from build123d import *

# Parameters (mm, degrees)
SKETCH_2_R               = 25
EXTRUDE_1_DEPTH          = 6
SKETCH_3_R               = 30
EXTRUDE_2_DEPTH          = 2
EXTRUDE_START            = 2
SKETCH_4_R               = 30
EXTRUDE_4_DEPTH          = 2
CUT_EXTRUDE_1_DEPTH      = 44.588989435
CUT_EXTRUDE_1_DEPTH_BACK = 44.588989435
SKETCH_5_R               = 20
CUT_EXTRUDE_3_DEPTH      = 44.588989435
CUT_EXTRUDE_3_DEPTH_BACK = 44.588989435
SKETCH_7_R               = 1.25


with BuildPart() as part:
    # 스케치2 → 보스-돌출1 (new body)
    with BuildSketch(Plane.XY):
        Circle(SKETCH_2_R)
    extrude(amount=EXTRUDE_1_DEPTH)

    # 스케치3 → 보스-돌출2 (add)
    with BuildSketch(Plane.XY.offset(6)):
        Circle(SKETCH_3_R)
    extrude(amount=EXTRUDE_2_DEPTH)

    # 스케치4 → 보스-돌출4 (add)
    with BuildSketch(Plane(origin=(0, 0, 0), x_dir=(-1, 0, 0), z_dir=(0, 0, -1)).offset(EXTRUDE_START)):
        with Locations(Location((0, 0, 0), (0, 0, 180))):
            Circle(SKETCH_4_R)
    extrude(amount=-EXTRUDE_4_DEPTH)

    # 스케치5 → 컷-돌출1 (cut, two sides: drawn at the far end of the back side and taken through both)
    with BuildSketch(Plane(origin=(0, 0, -2), x_dir=(-1, 0, 0), z_dir=(0, 0, -1)).offset(-CUT_EXTRUDE_1_DEPTH_BACK)):
        Circle(SKETCH_5_R)
    extrude(amount=CUT_EXTRUDE_1_DEPTH + CUT_EXTRUDE_1_DEPTH_BACK, mode=Mode.SUBTRACT)

    # 스케치7 → 컷-돌출3 (cut, two sides: drawn at the far end of the back side and taken through both)
    with BuildSketch(Plane.XY.offset(8).offset(-CUT_EXTRUDE_3_DEPTH_BACK)):
        with Locations((-27, 0)):
            Circle(SKETCH_7_R)
    extrude(amount=CUT_EXTRUDE_3_DEPTH + CUT_EXTRUDE_3_DEPTH_BACK, mode=Mode.SUBTRACT)


solid = part.part
Input: part model. Units: mm. Frame: model coordinates. A direction names the side the tool comes from. Round coordinates to 2 decimals unless told otherwise and drop trailing zeros. Order: outer loops, then holes, each group sorted by start corner. A loop starts at its lowest first (then second) coordinate and runs counter-clockwise, first axis right, second up. Notation, with made-up numbers: (58, 72.25) - (99, 72.25) arc R29 cw to (99, 107.25) - close; hole circle Ø1 at (61, 45). An arc over 180 degrees is marked (long way). Answer as a JSON object with one key per item and string values. Group by question number.
(1) Pin query (flat end, axial travel): P1, Ø2, axis at y = 24, z = 4.5, coming from the -X side; P2, Ø6, axis at x = -7.5, z = 1, coming from the +Y side; P3, Ø3, axis at x = -7.5, z = 0, coming from the -Y side. Return the tip coordinate at first contact, or that it passes through.
(2) Cut plane D-D (x = -27). Return loops of the section in (y, z), then the cut area to 3 significant figures.
(3) Cut plane C-C (z = 2). Return loops of the section in (x, y), then the cut area to 3 significant figures.
(4) Reachability of faces 1 (the face through (20, -6, 8)), 2 (the face through (-18, 18, 0)) from +Z, -Z, +X, -X, +Y, -Y: full face, straight path, thin tool, end or side. Return the list, or none.
(5) Cut plane A-A (y = 0). Return loops of the section in (x, z).
(6) Draft query along Z for faces 3 (the face through (-18, -18, 6)), 4 (the face through (20, 6, -2)), 5 (the face through (16.128, -25.296, -1.014)). Return one class per face: released by +Z, released by -Z, zero draft, split by the parting line, or undercut.
(7) Material intervals for probe 1 along Z at (x, y) = (-25, 13.5); probe 2 along Y at (x, z) = (0, 3.5); probe 3 along Y at (x, z) = (-16.5, 4.25), sorted ascending. Write a range as from..to.
(8) Cut plane B-B (x = 0). Return loops of the section in (y, z), then the cut area to 3 significant figures.
Here are the results:
{
 "1": {"P1": "stops at x = -9.8", "P2": "stops at y = 29.63", "P3": "stops at y = -29.39"},
 "2": {"outline": "(-13.08, -2) - (-1.25, -2) - (-1.25, 0) - (-13.08, 0) - close; (-13.08, 6) - (-1.25, 6) - (-1.25, 8) - (-13.08, 8) - close; (1.25, -2) - (13.08, -2) - (13.08, 0) - (1.25, 0) - close; (1.25, 6) - (13.08, 6) - (13.08, 8) - (1.25, 8) - close", "area": "94.6 mm^2"},
 "3": {"outline": "circle Ø50 at (0, 0); hole circle Ø40 at (0, 0)", "area": "707 mm^2"},
 "4": {"face 1": "+Z, +X, -X, +Y, -Y", "face 2": "none"},
 "5": {"outline": "(-30, -2) - (-28.25, -2) - (-28.25, 0) - (-30, 0) - close; (-30, 6) - (-28.25, 6) - (-28.25, 8) - (-30, 8) - close; (-25.75, -2) - (-20, -2) - (-20, 8) - (-25.75, 8) - (-25.75, 6) - (-25, 6) - (-25, 0) - (-25.75, 0) - close; (20, -2) - (30, -2) - (30, 0) - (25, 0) - (25, 6) - (30, 6) - (30, 8) - (20, 8) - close"},
 "6": {"face 3": "undercut", "face 4": "released by -Z", "face 5": "zero draft"},
 "7": {"probe 1": "z = -2..0, 6..8", "probe 2": "y = -25..-20, 20..25", "probe 3": "y = -18.78..-11.3, 11.3..18.78"},
 "8": {"outline": "(-30, -2) - (-20, -2) - (-20, 8) - (-30, 8) - (-30, 6) - (-25, 6) - (-25, 0) - (-30, 0) - close; (20, -2) - (30, -2) - (30, 0) - (25, 0) - (25, 6) - (30, 6) - (30, 8) - (20, 8) - close", "area": "140 mm^2"}
}
